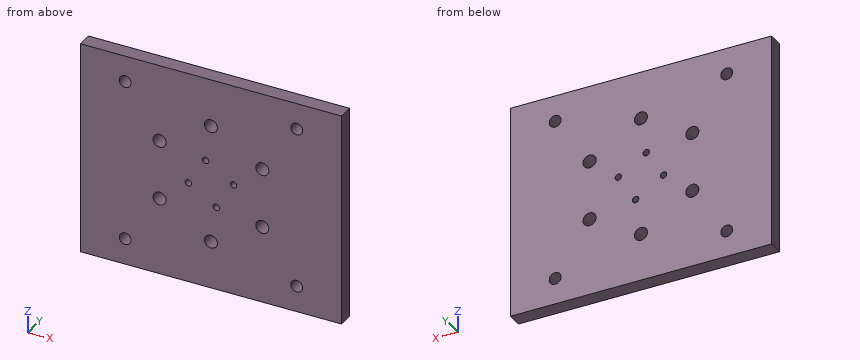
from build123d import *

# Parameters (mm, degrees)
SKETCH2_W            = 110
SKETCH2_H            = 90
BOSS_EXTRUDE1_DEPTH  = 6.35
SKETCH3_R            = 2.5
MOUNTING_HOLES_DEPTH = 143.268487375
CUT_EXTRUDE1_REACH   = 144.268
SKETCH4_R            = 2.75
CUT_EXTRUDE2_REACH   = 144.268
SKETCH5_R            = 1.355


with BuildPart() as part:
    # Sketch2 → Boss-Extrude1 (new body)
    with BuildSketch(Plane(origin=(0, 0, 0), x_dir=(1, 0, 0), z_dir=(0, 1, 0))):
        with Locations((55, 45)):
            Rectangle(SKETCH2_W, SKETCH2_H)
    extrude(amount=BOSS_EXTRUDE1_DEPTH)

    # Sketch3 → Mounting Holes (cut, through all)
    with BuildSketch(Plane(origin=(0, 6.35, 0), x_dir=(1, 0, 0), z_dir=(0, 1, 0))):
        with Locations(Location((18.85, 79, 0), (0, 0, 270))):
            Circle(SKETCH3_R)
        with Locations(Location((18.85, 11, 0), (0, 0, 90))):
            Circle(SKETCH3_R)
        with Locations(Location((91.15, 11, 0), (0, 0, 270))):
            Circle(SKETCH3_R)
        with Locations(Location((91.15, 79, 0), (0, 0, 90))):
            Circle(SKETCH3_R)
    extrude(amount=-MOUNTING_HOLES_DEPTH, mode=Mode.SUBTRACT)

    # Sketch4 → Cut-Extrude1 (cut, up to next)
    with BuildSketch(Plane(origin=(0, 6.35, 0), x_dir=(1, 0, 0), z_dir=(0, 1, 0)), mode=Mode.PRIVATE) as cut_extrude1_sk1:
        with Locations(Location((55, 70, 0), (0, 0, 270))):
            Circle(SKETCH4_R)
    cut_extrude1_tool1 = extrude(cut_extrude1_sk1.sketch, amount=-CUT_EXTRUDE1_REACH, mode=Mode.PRIVATE) & part.part
    # Sketch4 → Cut-Extrude1 (cut, up to next)
    with BuildSketch(Plane(origin=(0, 6.35, 0), x_dir=(1, 0, 0), z_dir=(0, 1, 0)), mode=Mode.PRIVATE) as cut_extrude1_sk2:
        with Locations(Location((76.650635095, 57.5, 0), (0, 0, 270))):
            Circle(SKETCH4_R)
    cut_extrude1_tool2 = extrude(cut_extrude1_sk2.sketch, amount=-CUT_EXTRUDE1_REACH, mode=Mode.PRIVATE) & part.part
    # Sketch4 → Cut-Extrude1 (cut, up to next)
    with BuildSketch(Plane(origin=(0, 6.35, 0), x_dir=(1, 0, 0), z_dir=(0, 1, 0)), mode=Mode.PRIVATE) as cut_extrude1_sk3:
        with Locations(Location((76.650635095, 32.5, 0), (0, 0, 270))):
            Circle(SKETCH4_R)
    cut_extrude1_tool3 = extrude(cut_extrude1_sk3.sketch, amount=-CUT_EXTRUDE1_REACH, mode=Mode.PRIVATE) & part.part
    # Sketch4 → Cut-Extrude1 (cut, up to next)
    with BuildSketch(Plane(origin=(0, 6.35, 0), x_dir=(1, 0, 0), z_dir=(0, 1, 0)), mode=Mode.PRIVATE) as cut_extrude1_sk4:
        with Locations(Location((55, 20, 0), (0, 0, 270))):
            Circle(SKETCH4_R)
    cut_extrude1_tool4 = extrude(cut_extrude1_sk4.sketch, amount=-CUT_EXTRUDE1_REACH, mode=Mode.PRIVATE) & part.part
    # Sketch4 → Cut-Extrude1 (cut, up to next)
    with BuildSketch(Plane(origin=(0, 6.35, 0), x_dir=(1, 0, 0), z_dir=(0, 1, 0)), mode=Mode.PRIVATE) as cut_extrude1_sk5:
        with Locations(Location((33.349364905, 32.5, 0), (0, 0, 270))):
            Circle(SKETCH4_R)
    cut_extrude1_tool5 = extrude(cut_extrude1_sk5.sketch, amount=-CUT_EXTRUDE1_REACH, mode=Mode.PRIVATE) & part.part
    # Sketch4 → Cut-Extrude1 (cut, up to next)
    with BuildSketch(Plane(origin=(0, 6.35, 0), x_dir=(1, 0, 0), z_dir=(0, 1, 0)), mode=Mode.PRIVATE) as cut_extrude1_sk6:
        with Locations(Location((33.349364905, 57.5, 0), (0, 0, 270))):
            Circle(SKETCH4_R)
    cut_extrude1_tool6 = extrude(cut_extrude1_sk6.sketch, amount=-CUT_EXTRUDE1_REACH, mode=Mode.PRIVATE) & part.part
    add(cut_extrude1_tool1.solids().sort_by_distance((55, 6.35, -70))[0], mode=Mode.SUBTRACT)
    add(cut_extrude1_tool2.solids().sort_by_distance((76.650635, 6.35, -57.5))[0], mode=Mode.SUBTRACT)
    add(cut_extrude1_tool3.solids().sort_by_distance((76.650635, 6.35, -32.5))[0], mode=Mode.SUBTRACT)
    add(cut_extrude1_tool4.solids().sort_by_distance((55, 6.35, -20))[0], mode=Mode.SUBTRACT)
    add(cut_extrude1_tool5.solids().sort_by_distance((33.349365, 6.35, -32.5))[0], mode=Mode.SUBTRACT)
    add(cut_extrude1_tool6.solids().sort_by_distance((33.349365, 6.35, -57.5))[0], mode=Mode.SUBTRACT)

    # Sketch5 → Cut-Extrude2 (cut, up to next)
    with BuildSketch(Plane(origin=(0, 6.35, 0), x_dir=(1, 0, 0), z_dir=(0, 1, 0)), mode=Mode.PRIVATE) as cut_extrude2_sk1:
        with Locations(Location((64.516169974, 42.748034189, 0), (0, 0, 270))):
            Circle(SKETCH5_R)
    cut_extrude2_tool1 = extrude(cut_extrude2_sk1.sketch, amount=-CUT_EXTRUDE2_REACH, mode=Mode.PRIVATE) & part.part
    # Sketch5 → Cut-Extrude2 (cut, up to next)
    with BuildSketch(Plane(origin=(0, 6.35, 0), x_dir=(1, 0, 0), z_dir=(0, 1, 0)), mode=Mode.PRIVATE) as cut_extrude2_sk2:
        with Locations(Location((45.483830025, 47.251965809, 0), (0, 0, 270))):
            Circle(SKETCH5_R)
    cut_extrude2_tool2 = extrude(cut_extrude2_sk2.sketch, amount=-CUT_EXTRUDE2_REACH, mode=Mode.PRIVATE) & part.part
    # Sketch5 → Cut-Extrude2 (cut, up to next)
    with BuildSketch(Plane(origin=(0, 6.35, 0), x_dir=(1, 0, 0), z_dir=(0, 1, 0)), mode=Mode.PRIVATE) as cut_extrude2_sk3:
        with Locations(Location((57.251965809, 54.516169974, 0), (0, 0, 270))):
            Circle(SKETCH5_R)
    cut_extrude2_tool3 = extrude(cut_extrude2_sk3.sketch, amount=-CUT_EXTRUDE2_REACH, mode=Mode.PRIVATE) & part.part
    # Sketch5 → Cut-Extrude2 (cut, up to next)
    with BuildSketch(Plane(origin=(0, 6.35, 0), x_dir=(1, 0, 0), z_dir=(0, 1, 0)), mode=Mode.PRIVATE) as cut_extrude2_sk4:
        with Locations(Location((52.74803419, 35.483830024, 0), (0, 0, 270))):
            Circle(SKETCH5_R)
    cut_extrude2_tool4 = extrude(cut_extrude2_sk4.sketch, amount=-CUT_EXTRUDE2_REACH, mode=Mode.PRIVATE) & part.part
    add(cut_extrude2_tool1.solids().sort_by_distance((64.51617, 6.35, -42.748034))[0], mode=Mode.SUBTRACT)
    add(cut_extrude2_tool2.solids().sort_by_distance((45.48383, 6.35, -47.251966))[0], mode=Mode.SUBTRACT)
    add(cut_extrude2_tool3.solids().sort_by_distance((57.251966, 6.35, -54.51617))[0], mode=Mode.SUBTRACT)
    add(cut_extrude2_tool4.solids().sort_by_distance((52.748034, 6.35, -35.48383))[0], mode=Mode.SUBTRACT)


solid = part.part
Design review of the part built by this model. Coordinates are the model's own, in mm. Round coordinates to 2 decimals unless told otherwise and drop trailing zeros. Write each loop counter-clockwise with the first axis right and the second up, starting at its lowest first coordinate (ties: lowest second). Pieces come first, ordered by that corner, then holes. Notation, with made-up numbers: (46, -16.75) -> (96, -16.75) arc R10 ccw to (96, -4.75) -> close; hole circle Ø11 at (-8.5, 88.5). An arc over 180 degrees is marked (long way). One line per question, with ' | ' between items.
(1) Take a section at D-D, the plane y = 2. State how many separate pieces and enclosed holes the cut face has, and give its area (3 significant figures).
Result sheet:
separate pieces: 1 | enclosed holes: 14 | area: 9,660 mm2
(2) Take a section at B-B, the plane z = -79. State the section outline as (x, y) points, and give its area (3 significant figures).
Result sheet:
outline: (0, 0) -> (16.35, 0) -> (16.35, 6.35) -> (0, 6.35) -> close; (21.35, 0) -> (88.65, 0) -> (88.65, 6.35) -> (21.35, 6.35) -> close; (93.65, 0) -> (110, 0) -> (110, 6.35) -> (93.65, 6.35) -> close | area: 635 mm2
(3) Take a section at A-A, the plane x = 91.15. State the section outline as (y, z) points, and give its area (3 significant figures).
Result sheet:
outline: (0, -90) -> (6.35, -90) -> (6.35, -81.5) -> (0, -81.5) -> close; (0, -76.5) -> (6.35, -76.5) -> (6.35, -13.5) -> (0, -13.5) -> close; (0, -8.5) -> (6.35, -8.5) -> (6.35, 0) -> (0, 0) -> close | area: 508 mm2
(4) Take a section at C-C, the plane z = -20. State the section outline as (x, y) points, and give its area (3 significant figures).
Result sheet:
outline: (0, 0) -> (52.25, 0) -> (52.25, 6.35) -> (0, 6.35) -> close; (57.75, 0) -> (110, 0) -> (110, 6.35) -> (57.75, 6.35) -> close | area: 664 mm2
(5) Insertion check: P1, Ø12, axis at x = 49.5, z = -48.5, coming from the -Y side. The pin has a flat end and moves straight along its axis. Give the tip position at first contact, or say it passes through.
Result sheet:
P1: y = 0
(6) Wall thickness on line 1 (X direction, y = 2.25, z = -32.5); line 2 (Z direction, x = 18, y = 5.75); line 3 (X direction, y = 5.25, z = -79.5): over which ranges is each line inside the solid? List them lowest first. Write a range as [from, to].
Result sheet:
line 1: [0, 30.6], [36.1, 73.9], [79.4, 110] | line 2: [-90, -81.35], [-76.65, -13.35], [-8.65, 0] | line 3: [0, 16.4], [21.3, 88.7], [93.6, 110]
